The listing builds one solid part. Answer for the finished solid, in the listing's coordinates (mm). Face numbers are marked on the shaded views. Round coordinates to 2 decimals unless told otherwise and drop trailing zeros. Loops run counter-clockwise (first coordinate to the right, second up) from the corner with the lowest first, then second, coordinate; pieces in that order, holes last. Notation, with made-up numbers: (44.25, -24) - (64.25, -24) arc R20 ccw to (64.25, 6) - close; hole circle Ø6 at (58.5, 78.5). An arc over 180 degrees is marked (long way). One line per item, written item: value.
```python
from build123d import *

# Parameters (mm, degrees)
FILLET3_R           = 0.8
FILLET4_R           = 1
SKETCH6_R           = 2.45
BOSS_EXTRUDE2_DEPTH = 2.8
CHAMFER2_SIZE       = 9.05
SKETCH9_R           = 1.95


with BuildPart() as part:
    # Sketch1 → Revolve1 (revolve)
    with BuildSketch(Plane.XY, mode=Mode.PRIVATE) as revolve1_sk:
        Polygon((0, 3.363206456), (-11.5, 3.363206456), (-11.5, -1.676793544), (0, -1.676793544), (0, 0.423206456), (-9.5, 0.423206456), (-9.5, 3.163206456), (0, 3.163206456), align=None)
    revolve(revolve1_sk.sketch.rotate(Axis((0, 2.051889918, 0), (0, -1, 0)), 270), axis=Axis((0, 2.051889918, 0), (0, -1, 0)))

    # Fillet3
    fillet3_edges = [part.edges().sort_by_distance(p)[0] for p in [
        (0, 0.423206456, -9.5),
    ]]
    fillet(fillet3_edges, radius=FILLET3_R)

    # Fillet4
    fillet4_edges = [part.edges().sort_by_distance(p)[0] for p in [
        (0, 3.163206456, -9.5),
    ]]
    fillet(fillet4_edges, radius=FILLET4_R)

    # Sketch6 → Boss-Extrude2 (add)
    with BuildSketch(Plane.XZ.offset(1.676793544)):
        with Locations(Location((0, 0, 0), (0, 0, 270))):
            Circle(SKETCH6_R)
    extrude(amount=BOSS_EXTRUDE2_DEPTH)

    # Chamfer2
    # the kernel refuses this chamfer: 9.05 mm, written as the material it adds along each edge
    with BuildSketch(Plane(origin=(0, -1.676793544, 0), x_dir=(0, 0, -1), z_dir=(-1, 0, 0))) as chamfer2_piece_1_section:
        Polygon((2.45 + CHAMFER2_SIZE, 0), (2.45, CHAMFER2_SIZE), (2.45, 0), align=None)
    chamfer2_piece_1 = revolve(axis=Axis((0, -1.676793544, 0), (0, -1, 0)), mode=Mode.PRIVATE)
    chamfer2_piece_1 = chamfer2_piece_1 & Plane(origin=(0, -3.007193491, 0), x_dir=(0, 0, 1), z_dir=(0, -1, 0)) * Cylinder(11.5, 46, mode=Mode.PRIVATE)
    chamfer2_piece_1 = split(chamfer2_piece_1, bisect_by=Plane(origin=(0, -4.476793544, 10.030399947), z_dir=(0, 1, 0)), keep=Keep.TOP, mode=Mode.PRIVATE)
    add(chamfer2_piece_1)

    # Cut-Sweep1: sweep along a path in Sketch10
    with BuildLine(Plane.XY) as cut_sweep1_path:
        Line((0, 0.423206456), (0, 0.323206456))
        ThreePointArc((0, 0.323206456), (0.732233047, -1.444560497), (2.5, -2.176793544))
        Line((2.5, -2.176793544), (11.5, -2.176793544))
    # Sketch9 → Cut-Sweep1 (sweep, cut)
    with BuildSketch(Plane(origin=(0, 0.423206456, 0), x_dir=(1, 0, 0), z_dir=(0, 1, 0))):
        Circle(SKETCH9_R)
    sweep(path=cut_sweep1_path.line, mode=Mode.SUBTRACT)


solid = part.part
```
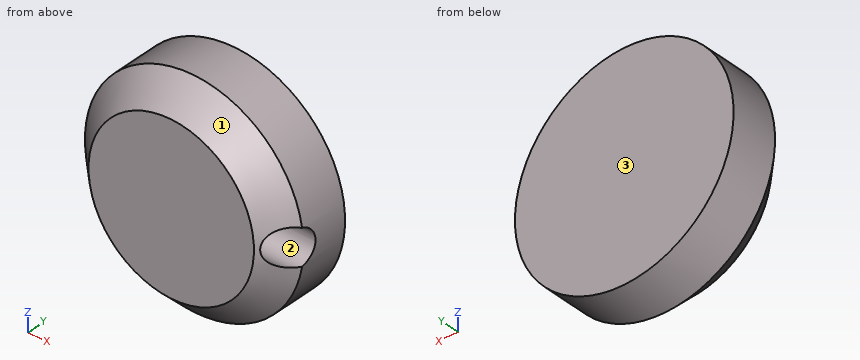
1) Each of these flat-tipped pins is pushed along its axis until it touches: pin 1 Ø1 at (y, z) = (-1.5, -2.5) entering from +X; pin 2 Ø3 at (x, y) = (8.5, -2.5) entering from +Z. Where does it stop, or does it pass through?
Final values:
pin 1: x = 11.32
pin 2: z = 8.93
2) A cutting plane is placed at C-C on y = 2.5. Give the vertices of the cut face in (x, z), and give its area (3 significant figures).
Final values:
outline: circle Ø23 at (0, 0); hole circle Ø18.88 at (0, 0)
area: 135 mm2
3) A cutting plane is placed at B-B on x = 5. Give the number of separate pieces and of enclosed holes in the cut face, and give its area (3 significant figures).
Final values:
separate pieces: 1
enclosed holes: 2
area: 98.1 mm2
4) Consider L1, parallel to Y at x = 4.5, z = 0; L2, parallel to X at y = 1.8, z = 0; L3, parallel to Y at x = 9, z = 1. Determine where each line is inside the solid, lowest interval first.
Final values:
L1: -4.48 to -4.13, -0.23 to 0.42, 3.16 to 3.36
L2: -11.5 to -9.5, 9.5 to 11.5
L3: -4.12 to -3.85, -0.5 to 0.51, 2.99 to 3.36
5) A cutting plane is placed at A-A on z = 0. Give the vertices of the cut face in (x, y).
Final values:
outline: (-11.5, -1.68) - (-8.7, -4.48) - (8.7, -4.48) - (9.05, -4.13) - (2.5, -4.13) arc R4.45 cw to (-1.95, 0.32) - (-1.95, 0.42) - (-8.7, 0.42) arc R0.8 cw to (-9.5, 1.22) - (-9.5, 2.16) arc R1 cw to (-8.5, 3.16) - (8.5, 3.16) arc R1 cw to (9.5, 2.16) - (9.5, 1.22) arc R0.8 cw to (8.7, 0.42) - (1.95, 0.42) - (1.95, 0.32) arc R0.55 ccw to (2.5, -0.23) - (11.5, -0.23) - (11.5, 3.36) - (-11.5, 3.36) - close
6) For a pull along Y with two mould halves and no side action, classify the marked faces 1, 2 and 3 as released by +Y, released by -Y, zero draft, split by the parting line, or undercut.
Final values:
face 1: released by -Y
face 2: undercut
face 3: released by +Y
